Read the model definition and answer for the solid it produces. Units are mm, in the model's axes. Round coordinates to 2 decimals unless told otherwise and drop trailing zeros. Order: outer loops, then holes, each group sorted by start corner. A loop starts at its lowest first (then second) coordinate and runs counter-clockwise, first axis right, second up. Notation, with made-up numbers: M -28.5,49.5 L 7.5,49.5 A20 ccw 7.5,68.5 Z; hole C -38,60.25 d6. An arc over 180 degrees is marked long. Answer as CSV lines item,"result".
```python
from build123d import *

# Parameters (mm, degrees)
F1_DEPTH = 6.35


with BuildPart() as f1:
    # F0 (on Top) → F1 (new body)
    with BuildSketch(Plane.XY):
        with BuildLine():
            Line((19.963766, 85.768253), (33.883162, 82.176149))
            ThreePointArc((33.883162, 82.176149), (37.161542, 71.464828), (28.771324, 64.042941))
            Line((28.771324, 64.042941), (13.19727, 68.062053))
            ThreePointArc((13.19727, 68.062053), (12.006678, 67.656763), (11.904457, 66.40324))
            ThreePointArc((11.904457, 66.40324), (18.129663, 59.81659), (25.941388, 55.221581))
            ThreePointArc((25.941388, 55.221581), (29.231866, 53.820261), (32.679028, 52.867364))
            ThreePointArc((32.679028, 52.867364), (35.880834, 52.556283), (39.06069, 53.042952))
            ThreePointArc((39.06069, 53.042952), (42.426036, 54.19472), (45.53752, 55.918317))
            ThreePointArc((45.53752, 55.918317), (50.903851, 58.755448), (56.458104, 61.204344))
            ThreePointArc((56.458104, 61.204344), (67.635189, 64.081109), (79.146661, 64.911172))
            ThreePointArc((79.146661, 64.911172), (126.658925, 66.093141), (174.185872, 66.132732))
            ThreePointArc((174.185872, 66.132732), (186.146195, 65.881821), (198.048443, 64.678162))
            ThreePointArc((198.048443, 64.678162), (202.485624, 63.728994), (206.752375, 62.184863))
            ThreePointArc((206.752375, 62.184863), (211.307712, 61.74472), (215.863049, 62.184863))
            ThreePointArc((215.863049, 62.184863), (225.059158, 73.821235), (215.863049, 85.457608))
            ThreePointArc((215.863049, 85.457608), (209.954904, 86.266057), (204.390645, 84.121577))
            ThreePointArc((204.390645, 84.121577), (198.525451, 82.399766), (192.482561, 81.478566))
            ThreePointArc((192.482561, 81.478566), (179.488338, 80.490153), (166.459054, 80.236152))
            ThreePointArc((166.459054, 80.236152), (126.883138, 79.702526), (87.307222, 80.236152))
            ThreePointArc((87.307222, 80.236152), (74.234888, 80.714226), (61.264478, 82.412139))
            ThreePointArc((61.264478, 82.412139), (54.766841, 84.972477), (48.795737, 88.594705))
            ThreePointArc((48.795737, 88.594705), (40.624685, 91.332134), (32.009568, 91.530554))
            ThreePointArc((32.009568, 91.530554), (24.876071, 90.45768), (18.504644, 87.074965))
            ThreePointArc((18.504644, 87.074965), (19.075081, 86.243925), (19.963766, 85.768253))
        make_face()
        Polygon((214.82671, 82.351932), (222.036342, 76.692745), (220.740158, 67.619426), (212.234342, 64.205295), (205.024709, 69.864482), (206.320893, 78.937801), align=None, mode=Mode.SUBTRACT)
    extrude(amount=F1_DEPTH)


solid = f1.part
```
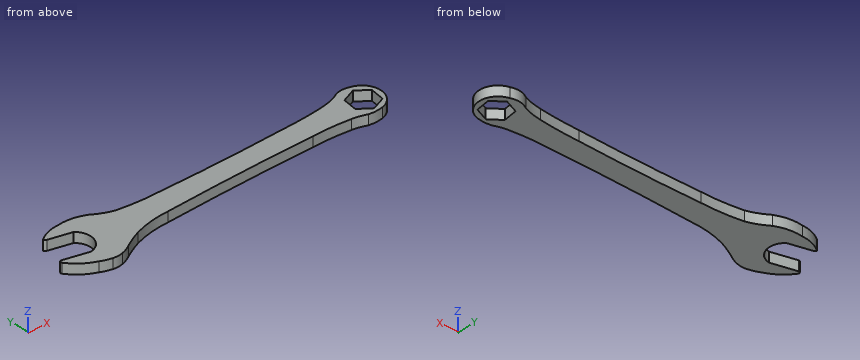
Item 1: A cutting plane is placed at D-D, the plane x = 83.5. Determine the outline of the cut face in (y, z).
Ans:
outline,"M 65.07,0 L 80.25,0 L 80.25,6.35 L 65.07,6.35 Z"
Item 2: A cutting plane is placed at A-A, the plane y = 72. Determine the outline of the cut face in (x, z).
Ans:
outline,"M 37.3,0 L 205.33,0 L 205.33,6.35 L 37.3,6.35 Z; M 221.37,0 L 224.92,0 L 224.92,6.35 L 221.37,6.35 Z"
Item 3: Find the intervals of material crossed by probe 1 along X at (y, z) = (72.5, 3.25); probe 2 along X at (y, z) = (70, 2.25); probe 3 along Y at (x, z) = (213.5, 1.25), in increasing order. Write a range as [from, to].
Ans:
probe 1,"[37.4, 205.4], [221.44, 224.99]"
probe 2,"[36.63, 205.04], [221.08, 224.43]"
probe 3,"[61.85, 64.71], [81.82, 86.15]"
Item 4: A cutting plane is placed at C-C, the plane x = 146. Determine the outline of the cut face in (y, z), and give its area (3 significant figures).
Ans:
outline,"M 66.25,0 L 79.83,0 L 79.83,6.35 L 66.25,6.35 Z"
area,"86.2 mm2"
Item 5: A flat-ended cylindrical pin translates along its axis: pin 1 (1 mm diameter, centred on y = 79, z = 1.5, fed in from +X). Find the tip coordinate at first contact, or state that the pin passes through.
Ans:
pin 1,"x = 224.11"
